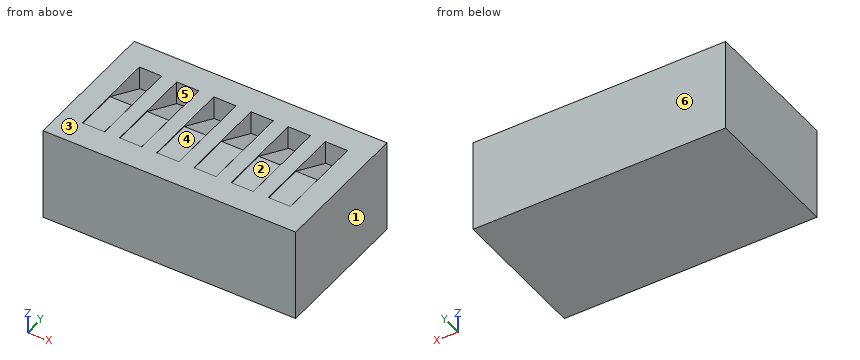
Autodesk Inventor part; units mm, degrees
ref_plane "YZ Plane" through (0, 0, 0) normal (1, 0, 0) x (0, 1, 0)
ref_plane "XZ Plane" through (0, 0, 0) normal (0, 1, 0) x (-1, 0, 0)
ref_plane "XY Plane" through (0, 0, 0) normal (0, 0, 1) x (1, 0, 0)
sketch "Sketch1" plane through (0, 0, 0) normal (0, 0, 1) x (1, 0, 0)
  line L0 (0, 0) -> (17.272, 0)
  line L1 (17.272, 0) -> (17.272, 9.7409)
  line L2 (17.272, 9.7409) -> (0, 9.7409)
  line L3 (0, 9.7409) -> (0, 0)
  dimension "d0" = 9.7409
  dimension "d1" = 17.272
extrude "Extrusion1" add sketch "Sketch1" along normal blind 6.3881
sketch "Sketch2" plane through (0, 0, 6.3881) normal (0, 0, 1) x (1, 0, 0)
  line L0 (0, 0) -> (0, 9.7409)
  line L1 (17.272, 0) -> (0, 0)
  line L2 (0, 9.7409) -> (17.272, 9.7409)
  line L3 (1.524, 7.9185) -> (3.048, 7.9185)
  line L4 (3.048, 7.9185) -> (3.048, 1.8225)
  line L5 (3.048, 1.8225) -> (1.524, 1.8224)
  line L6 (1.524, 1.8224) -> (1.524, 7.9185)
  line L7 (3.048, 7.9185) -> (3.048, 9.7409)
  line L8 (1.524, 1.8224) -> (1.524, 0)
  dimension "d4" = 1.524
  dimension "d5" = 6.096
  dimension "d7" = 1.524
extrude "Extrusion2" cut sketch "Sketch2" against normal blind 2.54 contours L6 L3 L4 L5
sketch "Sketch6" plane through (0, 0, 3.8481) normal (0, 0, 1) x (1, 0, 0)
  line L0 (1.524, 1.8224) -> (3.048, 1.8225)
  line L1 (3.048, 1.8225) -> (3.048, 7.9185)
  line L2 (3.048, 7.9185) -> (1.524, 7.9185)
  line L3 (1.524, 7.9185) -> (1.524, 1.8224)
  line L4 (1.5494, 7.9185) -> (3.0226, 7.9184)
  line L5 (3.0226, 7.9184) -> (3.0226, 1.8225)
  line L6 (3.0226, 1.8225) -> (1.5494, 1.8224)
  line L7 (1.5494, 1.8224) -> (1.5494, 7.9185)
  line L8 (1.5494, 4.8704) -> (1.524, 4.8705) construction
  line L9 (3.0226, 4.8704) -> (3.048, 4.8704) construction
  dimension "d38" = 0.0254
extrude "Extrusion6" add sketch "Sketch6" along normal blind 2.5146 contours L7 L2 L5 L0
sketch "Sketch7" plane through (3.0226, 1.8225, 3.8481) normal (1, 0, 0) x (0, 0, -1)
  line L0 (-2.5146, 6.096) -> (-2.5146, 0)
  line L1 (-2.5146, 6.096) -> (0, 6.096)
  line L2 (-0.9525, 6.096) -> (-2.5146, 2.921)
  point P0 (-2.54, 6.096)
  dimension "d41" = 3.175
  dimension "d42" = 1.5875
extrude "Extrusion7" cut sketch "Sketch7" against normal up to surface (1.4986 mm away)
pattern_linear "Rectangular Pattern5" count 6 spacing 2.54 along (1, 0, 0) of "Extrusion2"
pattern_linear "Rectangular Pattern6" count 6 spacing 2.54 along (1, 0, 0) of "Extrusion6", "Extrusion7"
properties part number "cRIO-FRC DIP Switch" material "ABS Plastic"
Verification items for the finished model (mm, model axes). Face numbers are marked on the shaded views. A direction names the side the tool comes from. Round coordinates to 2 decimals unless told otherwise and drop trailing zeros. Use one line per item in the form item = value.
1. Draft check along Y on the marked faces 3, 4, 5 and 6. Enter one of: pulls with the +Y half, pulls with the -Y half, needs draft (parallel to the pull), parting line crosses it, or undercut.
A:
face_3 = needs draft
face_4 = undercut
face_5 = undercut
face_6 = pulls with the +Y half
2. Gauge pin test, flat end, axial feed: pin 1 Ø1.7 at (x, z) = (4.5, 5) entering from -Y. Record the tip position at first contact, or that the pin passes through.
A:
pin_1 = 0
3. Section check A-A on z = 5.75. Give the number of separate pieces and of enclosed holes in the cut face, and give its area (3 significant figures).
A:
separate_pieces = 1
enclosed_holes = 6
area = 149 mm²
4. Access from +Z, -Z, +X, -X, +Y, -Y to the whole of each face (thin tool, end or side, straight path). Record for the marked faces 1 and 2.
A:
face_1 = +Z, -Z, +X, +Y, -Y
face_2 = +Z
5. Scan lines: probe 1 along Z at (x, y) = (2.5, 4.25); probe 2 along Z at (x, y) = (10.5, 6.75); probe 3 along Y at (x, z) = (10, 5.5). Record each from-to range of solid material in increasing order.
A:
probe_1 = 0 to 6.36
probe_2 = 0 to 5.38
probe_3 = 0 to 6.5, 7.92 to 9.74
